from build123d import *

# Parameters (mm, degrees)
SKETCH3_R          = 3
CUT_EXTRUDE1_DEPTH = 5


with BuildPart() as part:
    # Sketch1 → Revolve1 (revolve)
    with BuildSketch(Plane.XY, mode=Mode.PRIVATE) as revolve1_sk:
        Polygon((0, 0), (3.5, 0), (3.5, 2.8), (5.1, 2.8), (5.1, 14.8), (3.65, 14.8), (3.65, 17.9), (3.55, 17.9), (3.55, 19.9), (0, 19.9), align=None)
    revolve(revolve1_sk.sketch.rotate(Axis((0, 0, 0), (0, 1, 0)), 90), axis=Axis((0, 0, 0), (0, 1, 0)))

    # Sketch3 → Cut-Extrude1 (cut)
    with BuildSketch(Plane(origin=(0, 19.9, 0), x_dir=(1, 0, 0), z_dir=(0, 1, 0))):
        with Locations(Location((0, 0, 0), (0, 0, 270))):
            Circle(SKETCH3_R)
    extrude(amount=-CUT_EXTRUDE1_DEPTH, mode=Mode.SUBTRACT)


solid = part.part
Part model, mm, in its own coordinate system. A direction names the side the tool comes from. Give positions to 0.01 mm unless a question says otherwise; leave off trailing zeros. Loops run counter-clockwise (first coordinate to the right, second up) from the corner with the lowest first, then second, coordinate; pieces in that order, holes last.
(1) Band-saw the part on B-B (y = 16.5). Write the cut outline in (x, z), and give its area (3 significant figures).
Return value:
outline: circle Ø7.3 at (0, 0); hole circle Ø6 at (0, 0)
area: 13.6 mm2
(2) Band-saw the part on D-D (y = 12). Write the cut outline in (x, z), and give its area (3 significant figures).
Return value:
outline: circle Ø10.2 at (0, 0)
area: 81.7 mm2
(3) 3-axis set-ups, long thin cutter, end or side, ignore diameter. For faces 1 (the cylindrical face through (0.9, 17.43, 2.86)), 2 (the flat face through (-3, 19.9, 1)), 3 (the cylindrical face through (3.105, 1.42, -1.615)): which of +Z, -Z, +X, -X, +Y, -Y reach the whole face in a straight line?
Return value:
face 1: +Y
face 2: +Z, -Z, +X, -X, +Y
face 3: -Y
(4) Drill centre lines: line 1 along X through (y, z) = (16.1, 0); line 2 along Y through (x, z) = (3.5, -1.5); line 3 along X through (y, z) = (18.35, 0). Where is each one in solid material? Low to high.
Return value:
line 1: x = -3.65 to -3, 3 to 3.65
line 2: y = 2.8 to 14.8
line 3: x = -3.55 to -3, 3 to 3.55
(5) Pull direction X, two halves, no side cores. Call faces 4 (the flat face through (-3.5, 2.8, 1.1)), 5 (the cylindrical face through (-1.1, 16.37, -3.48)), 6 (the flat face through (0, 14.9, 0)): pulls with the +X half, pulls with the -X half, needs draft (parallel to the pull), parting line crosses it, or undercut.
Return value:
face 4: needs draft
face 5: parting line crosses it
face 6: undercut
(6) Pin check, flat tips, straight feed: pin 1 (3 mm diameter, centred on x = 3.5, y = 4.5, fed in from +Z); pin 2 (1 mm diameter, centred on y = 11, z = 3.5, fed in from -X). Stop position of each tip, or through.
Return value:
pin 1: stops at z = 4.69
pin 2: stops at x = -4.12
(7) Band-saw the part on A-A (z = 0). Write the cut outline in (x, y).
Return value:
outline: (-5.1, 2.8) - (-3.5, 2.8) - (-3.5, 0) - (3.5, 0) - (3.5, 2.8) - (5.1, 2.8) - (5.1, 14.8) - (3.65, 14.8) - (3.65, 17.9) - (3.55, 17.9) - (3.55, 19.9) - (3, 19.9) - (3, 14.9) - (-3, 14.9) - (-3, 19.9) - (-3.55, 19.9) - (-3.55, 17.9) - (-3.65, 17.9) - (-3.65, 14.8) - (-5.1, 14.8) - close
(8) Band-saw the part on C-C (x = 0). Write the cut outline in (y, z).
Return value:
outline: (0, -3.5) - (2.8, -3.5) - (2.8, -5.1) - (14.8, -5.1) - (14.8, -3.65) - (17.9, -3.65) - (17.9, -3.55) - (19.9, -3.55) - (19.9, -3) - (14.9, -3) - (14.9, 3) - (19.9, 3) - (19.9, 3.55) - (17.9, 3.55) - (17.9, 3.65) - (14.8, 3.65) - (14.8, 5.1) - (2.8, 5.1) - (2.8, 3.5) - (0, 3.5) - close
